from build123d import *

# Parameters (mm, degrees)
EXTRUDE_1_DEPTH          = 14
CUT_EXTRUDE_1_DEPTH      = 6
SKETCH_3_R               = 8
CUT_EXTRUDE_2_DEPTH      = 1
CUT_EXTRUDE_2_DEPTH_BACK = 29
SKETCH_4_R               = 6.5
CUT_EXTRUDE_3_DEPTH      = 29
SKETCH_5_R               = 1.75
CUT_EXTRUDE_4_DEPTH      = 16
SKETCH_6_R               = 1.75
CUT_EXTRUDE_5_DEPTH      = 16.0000001
SKETCH_11_R              = 1.5
CUT_EXTRUDE_6_DEPTH      = 29.0000001
CHAMFER_1_SIZE           = 1


with BuildPart() as part:
    # 草图1 → 凸台-拉伸1 (new body, symmetric)
    with BuildSketch(Plane.XY):
        with BuildLine():
            Line((9.797958971, -10), (53.366750419, -10))
            ThreePointArc((53.366750419, -10), (70.93867824, -4.934097522), (63.105828541, 11.591109915))
            Line((63.105828541, 11.591109915), (50.383677548, 15))
            Line((50.383677548, 15), (-27.565507431, 15))
            ThreePointArc((-27.565507431, 15), (-36.443659616, 9.602001064), (-35.73696059, -0.764317242))
            ThreePointArc((-35.73696059, -0.764317242), (-29.353950463, -5.559863718), (-21.371826468, -5.720427806))
            ThreePointArc((-21.371826468, -5.720427806), (-15.596757504, -5.725786931), (-10.787686266, -8.923330377))
            ThreePointArc((-10.787686266, -8.923330377), (-0.731228007, -13.98089073), (9.797958971, -10))
        make_face()
    extrude(amount=EXTRUDE_1_DEPTH, both=True)

    # 草图2 → 切除-拉伸1 (cut, symmetric)
    with BuildSketch(Plane.XY):
        with BuildLine():
            Line((-25.114071484, 15), (-25.880172402, 19.294363036))
            Line((-25.880172402, 19.294363036), (-38.301734179, 16.64803031))
            Line((-38.301734179, 16.64803031), (-39.057829244, 0.337979629))
            Line((-39.057829244, 0.337979629), (-36.873567525, -9.914677417))
            Line((-36.873567525, -9.914677417), (-21.991683498, -16.836179697))
            Line((-21.991683498, -16.836179697), (-15.8349094, -12.46162968))
            Line((-15.8349094, -12.46162968), (-10.787686266, -8.923330377))
            ThreePointArc((-10.787686266, -8.923330377), (-15.290702499, -2.479910341), (-23.059900609, -1.282255262))
            ThreePointArc((-23.059900609, -1.282255262), (-33.319731944, 5.694068268), (-25.114071484, 15))
        make_face()
    extrude(amount=CUT_EXTRUDE_1_DEPTH, both=True, mode=Mode.SUBTRACT)

    # 草图3 → 切除-拉伸2 (cut, two sides)
    with BuildSketch(Plane.XY.offset(14)) as cut_extrude_2_sk:
        Circle(SKETCH_3_R)
    extrude(amount=CUT_EXTRUDE_2_DEPTH, mode=Mode.SUBTRACT)
    extrude(cut_extrude_2_sk.sketch, amount=-CUT_EXTRUDE_2_DEPTH_BACK, mode=Mode.SUBTRACT)

    # 草图4 → 切除-拉伸3 (cut, through all)
    with BuildSketch(Plane.XY.offset(14)):
        with Locations((60, 0)):
            Circle(SKETCH_4_R)
    extrude(amount=-CUT_EXTRUDE_3_DEPTH, mode=Mode.SUBTRACT)

    # 草图5 → 切除-拉伸4 (cut, through all)
    with BuildSketch(Plane(origin=(0, 0, 0), x_dir=(1, 0, 0), z_dir=(0, 1, 0))):
        Circle(SKETCH_5_R)
    extrude(amount=CUT_EXTRUDE_4_DEPTH, mode=Mode.SUBTRACT)

    # 草图6 → 切除-拉伸5 (cut, through all)
    with BuildSketch(Plane(origin=(0, 0, 0), x_dir=(1, 0, 0), z_dir=(0, 1, 0))):
        with Locations((60, 0)):
            Circle(SKETCH_6_R)
    extrude(amount=CUT_EXTRUDE_5_DEPTH, mode=Mode.SUBTRACT)

    # 草图10 → M4 螺纹孔的螺纹孔钻头1 (revolve, cut)
    with BuildSketch(Plane(origin=(-25.114071484, 6.729295173, 14), x_dir=(0, -1, 0), z_dir=(1, 0, 0))):
        Polygon((0, 0), (0, 8.991420021), (1.65, 8), (1.65, 0.025), (1.675, 0), align=None)
    hole_wizard_m4_1 = revolve(axis=Axis((-25.114071484, 6.729295173, 20.35), (0, 0, -1)), mode=Mode.SUBTRACT)

    # 镜向1: M4 螺纹孔的螺纹孔钻头1 across plane
    add(hole_wizard_m4_1.mirror(Plane.XY), mode=Mode.SUBTRACT)

    # 草图11 → 切除-拉伸6 (cut, through all)
    with BuildSketch(Plane.XY.offset(14)):
        with Locations((-25.114071484, 6.729295173)):
            Circle(SKETCH_11_R)
    extrude(amount=-CUT_EXTRUDE_6_DEPTH, mode=Mode.SUBTRACT)

    # 倒角1
    chamfer_1_edges = [part.edges().sort_by_distance(p)[0] for p in [
        (-8, 0, 14),
        (-8, 0, -14),
        (53.5, 0, -14),
        (53.5, 0, 14),
    ]]
    chamfer(chamfer_1_edges, length=CHAMFER_1_SIZE)


solid = part.part
Build history of the part. All positions in model axes, mm. A direction names the side the tool comes from. Round coordinates to 2 decimals unless told otherwise and drop trailing zeros. Write each loop counter-clockwise with the first axis right and the second up, starting at its lowest first coordinate (ties: lowest second). Pieces come first, ordered by that corner, then holes. Notation, with made-up numbers: M -9,-37.75 L 44,-37.75 A20 ccw 44,-31.75 Z; hole C 45,10.5 d9. An arc over 180 degrees is marked long. Answer in a Markdown table with one row per item.
1. Mould opens along Y. For faces 1 (the face through (-36.37, 9.74, -9.94)), 2 (the face through (-0.89, -13.97, 0.2)), 3 (the face through (-26.613, 6.795, 0.083)), 4 (the face through (58.61, 9.55, 1.06)) say: +Y half, -Y half, draft (parallel to the pull), parting line (faces both ways), or undercut.
Geometry check:
| item | result |
|---|---|
| face 1 | parting line |
| face 2 | -Y half |
| face 3 | undercut |
| face 4 | draft |
2. Probe L1, parallel to X at y = 10.75, z = 0; L2, parallel to Z at x = -30.5, y = -2; L3, parallel to Y at x = 0, z = -5.25. List the from-to ranges inside material, lowest first. Write a range as [from, to].
Geometry check:
| item | result |
|---|---|
| L1 | [-32.34, -1.75], [1.75, 58.25], [61.75, 65.33] |
| L2 | [-14, -6], [6, 14] |
| L3 | [-14, -8], [8, 15] |
3. Saw through at B-B (z = 3.25). List the corners of the cut face in (x, y).
Geometry check:
| item | result |
|---|---|
| outline | M -25.11,15 A8.27 ccw long -23.06,-1.28 A10 cw -10.79,-8.92 A14 ccw 9.8,-10 L 53.37,-10 A12 ccw long 63.11,11.59 L 50.38,15 Z; hole C -25.11,6.73 d3; hole C 0,0 d16; hole C 60,0 d13 |
4. Saw through at C-C (x = 60). List the corners of the cut face in (y, z), and give its area (3 significant figures).
Geometry check:
| item | result |
|---|---|
| outline | M -12,-14 L -7.5,-14 L -6.5,-13 L -6.5,13 L -7.5,14 L -12,14 Z; M 6.5,-13 L 7.5,-14 L 12.42,-14 L 12.42,-1.75 L 6.5,-1.75 Z; M 6.5,1.75 L 12.42,1.75 L 12.42,14 L 7.5,14 L 6.5,13 Z |
| area | 297 mm2 |
5. Flat gauge pins, fed straight in: P1, Ø4.5, axis at x = 60, z = 0, coming from the +Y side; P2, Ø3, axis at y = -4.5, z = 3.5, coming from the +X side; P3, Ø3, axis at x = -6, z = 0.5, coming from the -Y side. Where does each tip first touch, or does it go through?
Geometry check:
| item | result |
|---|---|
| P1 | y = 13.03 |
| P2 | x = 71.62 |
| P3 | y = -13.26 |
6. Saw through at D-D (y = -3.25). State how many separate pieces and enclosed holes the cut face has, and give its area (3 significant figures).
Geometry check:
| item | result |
|---|---|
| separate pieces | 3 |
| enclosed holes | 0 |
| area | 1,980 mm2 |
7. Which spindle directions (+Z, -Z, +X, -X, +Y, -Y) get a long thin tool onto all of the face, cutting with end or side? Do faces 5 (the face through (1.617, 11.35, 0.67)), 6 (the face through (-15.195, -2.54, 0.084)), 7 (the face through (31, -10, 0)). Say none if no direction does.
Geometry check:
| item | result |
|---|---|
| face 5 | +Y |
| face 6 | -Y |
| face 7 | +Z, -Z, -Y |
8. Saw through at A-A (x = 0). List the corners of the cut face in (y, z), and give its area (4 significant figures).
Geometry check:
| item | result |
|---|---|
| outline | M -14,-14 L -9,-14 L -8,-13 L -8,13 L -9,14 L -14,14 Z; M 8,-13 L 9,-14 L 15,-14 L 15,-1.75 L 8,-1.75 Z; M 8,1.75 L 15,1.75 L 15,14 L 9,14 L 8,13 Z |
| area | 337.5 mm2 |
